from build123d import *

# Parameters (mm, degrees)
PAD_DEPTH    = 9
SKETCH001_W  = 47
SKETCH001_H  = 6
POCKET_DEPTH = 7


with BuildPart() as part:
    # Sketch → Pad (new body, symmetric)
    with BuildSketch(Plane.XZ):
        Polygon((-20.679492, 25.679492), (15.320508, 25.679492), (28, 13), (28, 0), (-28, 0), (-28, 13), align=None)
    extrude(amount=PAD_DEPTH, both=True)

    # Sketch001 (on Face1 of Pad) → Pocket (cut)
    with BuildSketch(Plane(origin=(0, 0, 25.679492), x_dir=(-1, 0, 0), z_dir=(0, 0, 1))):
        Rectangle(SKETCH001_W, SKETCH001_H)
    extrude(amount=-POCKET_DEPTH, mode=Mode.SUBTRACT)


solid = part.part
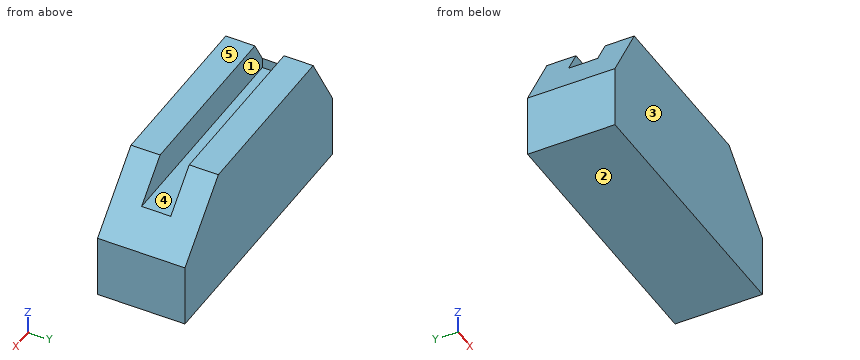
Work out the finished part from the listing and answer in its coordinate system (mm). Face numbers are marked on the shaded views. A direction names the side the tool comes from. Round coordinates to 2 decimals unless told otherwise and drop trailing zeros. Write each loop counter-clockwise with the first axis right and the second up, starting at its lowest first coordinate (ties: lowest second). Pieces come first, ordered by that corner, then holes.
1) The mould has two halves that part along Y. Classify the marked faces 3, 4 and 5: pulls with the +Y half, pulls with the -Y half, needs draft (parallel to the pull), parting line crosses it, or undercut.
2) A cutting plane is placed at D-D (z = 19.5). Give the vertices of the cut face in (x, y).
3) A cutting plane is placed at C-C (x = 16). Give the vertices of the cut face in (y, z).
4) Straight lines are drawn through the part: line 1 (Y direction, x = 20.5, z = 19.75); line 2 (Z direction, x = 18.5, y = 0.5); line 3 (X direction, y = -3.75, z = 21.5). For each, find the intervals that lie inside material, in ascending order.
5) A cutting plane is placed at A-A (y = 0.5). Give the vertices of the cut face in (x, z).
6) Given pin 1 Ø8 at (y, z) = (-1, 18) entering from +X; pin 2 Ø3 at (y, z) = (3.5, 15.5) entering from -X; pin 3 Ø4 at (x, y) = (21, -3) entering from -Z; pin 4 Ø1.1 at (y, z) = (0.5, 19.5) entering from +X, each flat-ended and moving along its own axis, determine where each tip first touches the part or whether it passes through.
7) A cutting plane is placed at B-B (z = 22.75). Give the vertices of the cut face in (x, y).
8) A tool of negligible diameter and unlimited length cuts with its end or side. For the marked faces 1 and 2, from which of +Z, -Z, +X, -X, +Y, -Y can it reach the whole face along a straight path? Write none if from no direction.
Completed:
1. face 3: pulls with the -Y half
1. face 4: undercut
1. face 5: needs draft
2. outline: (-24.25, -9) - (21.5, -9) - (21.5, -3) - (-23.5, -3) - (-23.5, 3) - (21.5, 3) - (21.5, 9) - (-24.25, 9) - close
3. outline: (-9, 0) - (9, 0) - (9, 25) - (3, 25) - (3, 18.68) - (-3, 18.68) - (-3, 25) - (-9, 25) - close
4. line 1: y = -9 to -3, 3 to 9
4. line 2: z = 0 to 18.68
4. line 3: x = -23.09 to 19.5
5. outline: (-28, 0) - (28, 0) - (28, 13) - (22.32, 18.68) - (-23.5, 18.68) - (-23.5, 20.79) - (-28, 13) - close
6. pin 1: stops at x = 27
6. pin 2: stops at x = -27.42
6. pin 3: stops at z = 0
6. pin 4: stops at x = -23.5
7. outline: (-22.37, -9) - (18.25, -9) - (18.25, -3) - (-22.37, -3) - close; (-22.37, 3) - (18.25, 3) - (18.25, 9) - (-22.37, 9) - close
8. face 1: +Z, +X
8. face 2: -Z, +X, -X, +Y, -Y
